from build123d import *

# Parameters (mm, degrees)
F4_DEPTH  = 30.001
F5_W      = 6
F5_H      = 7
F6_DEPTH  = 13
F7_W      = 38.173924
F7_H      = 20
F8_DEPTH  = 30.001
F9_W      = 3
F9_H      = 3
F10_DEPTH = 7
F11_DEPTH = 30.001


with BuildPart() as f1:
    # F0 (on Right) → F1 (revolve)
    with BuildSketch(Plane.YZ):
        with BuildLine():
            Line((-30, 0), (0, 0))
            ThreePointArc((0, 0), (-15, 15), (-30, 0))
        make_face()
    revolve(axis=Axis((0, -15, 0), (0, -1, 0)))

    # F3 (on offset) → F4 (cut, through all)
    with BuildSketch(Plane.XY.offset(15)):
        with BuildLine():
            Line((15, 0), (0, 0))
            Line((0, 0), (-15, 0))
            ThreePointArc((-15, 0), (0, -3), (15, 0))
        make_face()
    extrude(amount=-F4_DEPTH, mode=Mode.SUBTRACT)

    # F5 (on Front) → F6 (cut)
    with BuildSketch(Plane.XZ):
        Rectangle(F5_W, F5_H)
    extrude(amount=F6_DEPTH, mode=Mode.SUBTRACT)

    # F7 (on Front) → F8 (cut, through all)
    with BuildSketch(Plane.XZ):
        with Locations((0, -13.5)):
            Rectangle(F7_W, F7_H)
    extrude(amount=F8_DEPTH, mode=Mode.SUBTRACT)

    # F9 (on face) → F10 (cut)
    with BuildSketch(Plane(origin=(0, 0, -3.5), x_dir=(1, 0, 0), z_dir=(0, 0, -1))):
        with Locations((-4.5, 11.5)):
            Rectangle(F9_W, F9_H)
        with Locations((4.5, 11.5)):
            Rectangle(F9_W, F9_H)
    extrude(amount=-F10_DEPTH, mode=Mode.SUBTRACT)

    # F7 (on Front) → F11 (cut, through all)
    with BuildSketch(Plane.XZ):
        with Locations((0, -13.5)):
            Rectangle(F7_W, F7_H)
    extrude(amount=F11_DEPTH, mode=Mode.SUBTRACT)


solid = f1.part
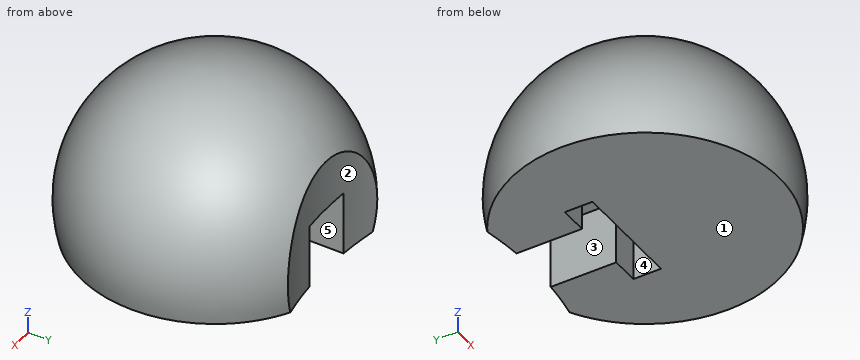
Here's how the part is built. I have some questions about the finished solid (model axes, mm). Face numbers are marked on the shaded views. A direction names the side the tool comes from. Coordinates: 2 decimals unless noted, no trailing zeros. Loops run counter-clockwise (first coordinate to the right, second up) from the corner with the lowest first, then second, coordinate; pieces in that order, holes last.
1. For the marked faces 4 and 5, which set-ups out of +Z, -Z, +X, -X, +Y, -Y let a thin tool reach every point of the face, with its end or its side?
2. Imagine slicing it at C-C, the plane x = -1.75. Please give me the cut outline in (y, z).
3. Imagine slicing it at D-D, the plane z = 4. Please give me the cut outline in (x, y), and give its area (3 significant figures).
4. If we mould it in two halves opening along X, with no side actions, what happens to the marked faces 1, 2 and 3? For each: pulls with the +X half, pulls with the -X half, needs draft (parallel to the pull), parting line crosses it, or undercut.
5. For P1, Ø5, axis at x = 2.5, y = -5.5, coming from the -Z side; P2, Ø6, axis at y = -15.5, z = 6.5, coming from the +X side; P3, Ø3.5, axis at y = -5.5, z = -1, coming from the +X side; P4, Ø7.5, axis at y = -8, z = 1, coming from the -X side, each with a flat end and sliding along its axis, tell me the tip position at first contact or that it passes through.
6. Imagine slicing it at B-B, the plane y = -12.25. Please give me the cut outline in (x, z), and give its area (3 significant figures).
7. I need wall thicknesses on L1, parallel to Y at x = -4.5, z = 1.75; L2, parallel to Y at x = -3.5, z = -1.75; L3, parallel to X at y = -25.5, z = 1.5. Which ranges of each line are inside material? Lowest first, please.
8. Imagine slicing it at A-A, the plane z = 2. Please give me the cut outline in (x, y).
Taken from the geometry:
1. face 4: -Z
1. face 5: -Z, +Y
2. outline: (-29.48, -3.5) - (-13, -3.5) - (-13, 3.5) - (-2.96, 3.5) - (-2.96, 8.77) arc R14.9 ccw to start
3. outline: (-7.02, -2.36) arc R14.46 ccw (long way) to (7.02, -2.36) arc R39 cw to start
3. area: 633 mm2
4. face 1: needs draft
4. face 2: undercut
4. face 3: undercut
5. P1: stops at z = -3.5
5. P2: stops at x = 14.58
5. P3: stops at x = 12.81
5. P4: stops at x = -14.63
6. outline: (-14.32, -3.5) - (-6, -3.5) - (-6, 3.5) - (6, 3.5) - (6, -3.5) - (14.32, -3.5) arc R14.75 ccw (long way) to start
6. area: 360 mm2
7. L1: y = -29.2 to -13, -10 to -2.74
7. L2: y = -29.48 to -13, -10 to -2.84
7. L3: x = -10.61 to 10.61
8. outline: (-7.64, -2.25) arc R14.87 ccw (long way) to (7.64, -2.25) arc R39 cw to (3, -2.88) - (3, -10) - (6, -10) - (6, -13) - (-6, -13) - (-6, -10) - (-3, -10) - (-3, -2.88) arc R39 cw to start
